Build history of the part. All positions in model axes, mm. Round coordinates to 2 decimals unless told otherwise and drop trailing zeros. Loops run counter-clockwise (first coordinate to the right, second up) from the corner with the lowest first, then second, coordinate; pieces in that order, holes last. Notation, with made-up numbers: (-27, 47) -> (21, 47) arc R23 cw to (21, 61) -> close; hole circle Ø2 at (46, -26.75). An arc over 180 degrees is marked (long way). Put each result on its own line as item: value. Start each with the question number.
```python
from build123d import *

# Parameters (mm, degrees)
CIRCLE_R         = 2.5
EXTRUDE_DEPTH    = 100
ARRAY_R          = 2.5
EXTRUDE001_DEPTH = 100
ARRAY001_R       = 2.5
EXTRUDE002_DEPTH = 100
ARRAY002_R       = 2.5
EXTRUDE003_DEPTH = 100
ARRAY003_R       = 2.5
EXTRUDE004_DEPTH = 100
SKETCH_R         = 57.5
PAD_DEPTH        = 4
SKETCH001_R      = 28.75
SKETCH001_R_2    = 25.75
PAD001_DEPTH     = 10


with BuildPart() as extrude_body:
    # Circle → Extrude (new body)
    with BuildSketch(Plane.XY):
        Circle(CIRCLE_R)
    extrude(amount=EXTRUDE_DEPTH)


with BuildPart() as extrude001:
    # Array → Extrude001 (new body)
    with BuildSketch(Plane(origin=(10, 0, 0), x_dir=(0, -1, 0), z_dir=(0, 0, -1))):
        Circle(ARRAY_R)
        with Locations((-7.071068, 2.928932)):
            Circle(ARRAY_R)
        with Locations((-10, 10)):
            Circle(ARRAY_R)
        with Locations((-7.071068, 17.071068)):
            Circle(ARRAY_R)
        with Locations((0, 20)):
            Circle(ARRAY_R)
        with Locations((7.071068, 17.071068)):
            Circle(ARRAY_R)
        with Locations((10, 10)):
            Circle(ARRAY_R)
        with Locations((7.071068, 2.928932)):
            Circle(ARRAY_R)
    extrude(amount=-EXTRUDE001_DEPTH)


with BuildPart() as extrude002:
    # Array001 → Extrude002 (new body)
    with BuildSketch(Plane(origin=(20, 0, 0), x_dir=(0, -1, 0), z_dir=(0, 0, -1))):
        Circle(ARRAY001_R)
        with Locations((-10, 2.679492)):
            Circle(ARRAY001_R)
        with Locations((-17.320508, 10)):
            Circle(ARRAY001_R)
        with Locations((-20, 20)):
            Circle(ARRAY001_R)
        with Locations((-17.320508, 30)):
            Circle(ARRAY001_R)
        with Locations((-10, 37.320508)):
            Circle(ARRAY001_R)
        with Locations((0, 40)):
            Circle(ARRAY001_R)
        with Locations((10, 37.320508)):
            Circle(ARRAY001_R)
        with Locations((17.320508, 30)):
            Circle(ARRAY001_R)
        with Locations((20, 20)):
            Circle(ARRAY001_R)
        with Locations((17.320508, 10)):
            Circle(ARRAY001_R)
        with Locations((10, 2.679492)):
            Circle(ARRAY001_R)
    extrude(amount=-EXTRUDE002_DEPTH)


with BuildPart() as extrude003:
    # Array002 → Extrude003 (new body)
    with BuildSketch(Plane(origin=(35, 0, 0), x_dir=(0, -1, 0), z_dir=(0, 0, -1))):
        Circle(ARRAY002_R)
        with Locations((-9.860639, 1.417746)):
            Circle(ARRAY002_R)
        with Locations((-18.922429, 5.556126)):
            Circle(ARRAY002_R)
        with Locations((-26.451235, 12.079874)):
            Circle(ARRAY002_R)
        with Locations((-31.83712, 20.460475)):
            Circle(ARRAY002_R)
        with Locations((-34.64375, 30.018981)):
            Circle(ARRAY002_R)
        with Locations((-34.64375, 39.981019)):
            Circle(ARRAY002_R)
        with Locations((-31.83712, 49.539525)):
            Circle(ARRAY002_R)
        with Locations((-26.451235, 57.920126)):
            Circle(ARRAY002_R)
        with Locations((-18.922429, 64.443874)):
            Circle(ARRAY002_R)
        with Locations((-9.860639, 68.582254)):
            Circle(ARRAY002_R)
        with Locations((0, 70)):
            Circle(ARRAY002_R)
        with Locations((9.860639, 68.582254)):
            Circle(ARRAY002_R)
        with Locations((18.922429, 64.443874)):
            Circle(ARRAY002_R)
        with Locations((26.451235, 57.920126)):
            Circle(ARRAY002_R)
        with Locations((31.83712, 49.539525)):
            Circle(ARRAY002_R)
        with Locations((34.64375, 39.981019)):
            Circle(ARRAY002_R)
        with Locations((34.64375, 30.018981)):
            Circle(ARRAY002_R)
        with Locations((31.83712, 20.460475)):
            Circle(ARRAY002_R)
        with Locations((26.451235, 12.079874)):
            Circle(ARRAY002_R)
        with Locations((18.922429, 5.556126)):
            Circle(ARRAY002_R)
        with Locations((9.860639, 1.417746)):
            Circle(ARRAY002_R)
    extrude(amount=-EXTRUDE003_DEPTH)


with BuildPart() as extrude004:
    # Array003 → Extrude004 (new body)
    with BuildSketch(Plane(origin=(45, 0, 0), x_dir=(0, -1, 0), z_dir=(0, 0, -1))):
        Circle(ARRAY003_R)
        with Locations((-9.356026, 0.983358)):
            Circle(ARRAY003_R)
        with Locations((-18.303149, 3.890454)):
            Circle(ARRAY003_R)
        with Locations((-26.450336, 8.594235)):
            Circle(ARRAY003_R)
        with Locations((-33.441517, 14.889123)):
            Circle(ARRAY003_R)
        with Locations((-38.971143, 22.5)):
            Circle(ARRAY003_R)
        with Locations((-42.797543, 31.094235)):
            Circle(ARRAY003_R)
        with Locations((-44.753485, 40.296219)):
            Circle(ARRAY003_R)
        with Locations((-44.753485, 49.703781)):
            Circle(ARRAY003_R)
        with Locations((-42.797543, 58.905765)):
            Circle(ARRAY003_R)
        with Locations((-38.971143, 67.5)):
            Circle(ARRAY003_R)
        with Locations((-33.441517, 75.110877)):
            Circle(ARRAY003_R)
        with Locations((-26.450336, 81.405765)):
            Circle(ARRAY003_R)
        with Locations((-18.303149, 86.109546)):
            Circle(ARRAY003_R)
        with Locations((-9.356026, 89.016642)):
            Circle(ARRAY003_R)
        with Locations((0, 90)):
            Circle(ARRAY003_R)
        with Locations((9.356026, 89.016642)):
            Circle(ARRAY003_R)
        with Locations((18.303149, 86.109546)):
            Circle(ARRAY003_R)
        with Locations((26.450336, 81.405765)):
            Circle(ARRAY003_R)
        with Locations((33.441517, 75.110877)):
            Circle(ARRAY003_R)
        with Locations((38.971143, 67.5)):
            Circle(ARRAY003_R)
        with Locations((42.797543, 58.905765)):
            Circle(ARRAY003_R)
        with Locations((44.753485, 49.703781)):
            Circle(ARRAY003_R)
        with Locations((44.753485, 40.296219)):
            Circle(ARRAY003_R)
        with Locations((42.797543, 31.094235)):
            Circle(ARRAY003_R)
        with Locations((38.971143, 22.5)):
            Circle(ARRAY003_R)
        with Locations((33.441517, 14.889123)):
            Circle(ARRAY003_R)
        with Locations((26.450336, 8.594235)):
            Circle(ARRAY003_R)
        with Locations((18.303149, 3.890454)):
            Circle(ARRAY003_R)
        with Locations((9.356026, 0.983358)):
            Circle(ARRAY003_R)
    extrude(amount=-EXTRUDE004_DEPTH)


with BuildPart() as cut004:
    # Sketch → Pad (new body)
    with BuildSketch(Plane.XY):
        Circle(SKETCH_R)
    extrude(amount=PAD_DEPTH)

    # Cut: cut Extrude004
    add(extrude004.part, mode=Mode.SUBTRACT)

    # Cut001: cut Extrude003
    add(extrude003.part, mode=Mode.SUBTRACT)

    # Cut002: cut Extrude002
    add(extrude002.part, mode=Mode.SUBTRACT)

    # Cut003: cut Extrude001
    add(extrude001.part, mode=Mode.SUBTRACT)

    # Cut004: cut Extrude body
    add(extrude_body.part, mode=Mode.SUBTRACT)


with BuildPart() as fusion:
    # Sketch001 → Pad001 (new body)
    with BuildSketch(Plane.XY):
        Circle(SKETCH001_R)
        Circle(SKETCH001_R_2, mode=Mode.SUBTRACT)
    extrude(amount=PAD001_DEPTH)

    # Fusion: union Cut004
    add(cut004.part)


solid = fusion.part
```
Item 1: Cut at C-C on z = 7.25. Write the cut outline in (x, y), then the cut area to 3 significant figures.
Item 2: Wall check: line 1 (Y direction, x = -4, z = 2.5); line 2 (X direction, y = -44.5, z = 2); line 3 (X direction, y = 38.5, z = 1). Give the ranges that are in metal, low to high. Write a range as from..to.
Item 3: Cut at A-A on x = 0. State how many separate pieces and enclosed holes the cut face has, then the cut area to 3 significant figures.
Item 4: Cut at D-D on y = 50.5. Write the cut outline in (x, z), then the cut area to 3 significant figures.
Item 5: Drop flat-ended pins along their axis: pin 1 (4 mm diameter, centred on y = -20, z = 5, fed in from -X); pin 2 (6 mm diameter, centred on x = -10, z = 3, fed in from +Y); pin 3 (1.5 mm diameter, centred on x = -31, y = 39, fed in from +Z). Give the stop position or say it passes through.
Item 6: Pull direction X, two halves, no side cores. Call faces 1 (the face through (-14.66, -45.18, 1.97)), 2 (the face through (31.104, -9.535, 1.972)): +X half, -X half, draft (parallel to the pull), parting line (faces both ways), or undercut.
Ans:
1. outline: circle Ø57.5 at (0, 0); hole circle Ø51.5 at (0, 0)
1. area: 514 mm2
2. line 1: y = -57.36..-47.15, -42.35..-36.94, -32.34..32.34, 36.94..42.35, 47.15..57.36
2. line 2: x = -36.41..-15.74, -12.08..-7.19, -2.22..2.22, 7.19..12.08, 15.74..36.41
2. line 3: x = -42.71..-24.96, -20.04..20.04, 24.96..42.71
3. separate pieces: 6
3. enclosed holes: 0
3. area: 396 mm2
4. outline: (-27.5, 0) -> (27.5, 0) -> (27.5, 4) -> (-27.5, 4) -> close
4. area: 220 mm2
5. pin 1: stops at x = -54.52
5. pin 2: stops at y = 57.07
5. pin 3: stops at z = 4
6. face 1: undercut
6. face 2: undercut
